Geometry check sheet. Reference: the model listing, model coordinates, mm. A direction names the side the tool comes from. Coordinates: 2 decimals unless noted, no trailing zeros. Order: outer loops, then holes, each group sorted by start corner. A loop starts at its lowest first (then second) coordinate and runs counter-clockwise, first axis right, second up.
```python
from build123d import *

# Parameters (mm, degrees)
SKETCH1_W           = 119.46432313
SKETCH1_H           = 3.175
BOSS_EXTRUDE1_DEPTH = 250


with BuildPart() as part:
    # Sketch1 → Boss-Extrude1 (new body)
    with BuildSketch(Plane.XY):
        Polygon((-4531.808395064, -128.147603784), (-4348.106631906, -144.21942553), (-4252.390993124, -156.337240533), (-4252.390993124, -153.162240533), (-4348.324803087, -141.01321004), (-4531.531675581, -124.984685617), align=None)
        with Locations((-4192.658831559, -154.749740533)):
            Rectangle(SKETCH1_W, SKETCH1_H)
    extrude(amount=-BOSS_EXTRUDE1_DEPTH)


solid = part.part
```
Item 1: Sectioned sample at A-A (z = -184.5). Record the cut outline in (x, y).
Item 2: Sectioned sample at B-B (x = -4214). Record the cut outline in (y, z).
Item 3: Sectioned sample at C-C (y = -137). Record the cut outline in (x, z), and give its area (3 significant figures).
Item 4: Thickness scan on line 1 along Y through (x, z) = (-4251, -224.5); line 2 along Y through (x, z) = (-4357, -89.5). Record the ranges inside material, lowest first.
Item 5: Tool access check on faces 1 (the face through (-4333, -144, 0)), 2 (the face through (-4193, -153.162, -123)). Record the directions out of +Z, -Z, +X, -X, +Y, -Y that give a thin tool (end or side, any length) a straight path to the whole face; none if there is none.
Geometry check:
1. outline: (-4531.81, -128.15) - (-4348.11, -144.22) - (-4252.39, -156.34) - (-4132.93, -156.34) - (-4132.93, -153.16) - (-4252.39, -153.16) - (-4348.32, -141.01) - (-4531.53, -124.98) - close
2. outline: (-156.34, -250) - (-153.16, -250) - (-153.16, 0) - (-156.34, 0) - close
3. outline: (-4430.63, -250) - (-4394.2, -250) - (-4394.2, 0) - (-4430.63, 0) - close
3. area: 9,110 mm2
4. line 1: y = -156.34 to -153.16
4. line 2: y = -143.44 to -140.25
5. face 1: +Z, +X, -X, +Y, -Y
5. face 2: +Z, -Z, +X, +Y
